For this review, take the finished solid that the model builds, in its own axes (mm). Give positions to 0.01 mm unless a question says otherwise; leave off trailing zeros. Order: outer loops, then holes, each group sorted by start corner. A loop starts at its lowest first (then second) coordinate and runs counter-clockwise, first axis right, second up.
Item 1: Consider section B-B (x = 2.5). Give the boundary of the cut face in (y, z).
Item 2: For probe 1 along X at (y, z) = (-22, 2.5); probe 2 along X at (y, z) = (-23, 2); probe 3 along X at (y, z) = (2.5, 11.75), list the stretches that pass through material, from the lowest coordinate up.
Item 3: Consider section C-C (y = -12). Give the boundary of the cut face in (x, z).
Item 4: Consider section A-A (y = 4.5). Give the boundary of the cut face in (x, z).
Item 5: Consider section D-D (z = 3.5). Give the boundary of the cut face in (x, y) (1 decimal), plus the area to 3 significant figures.
Item 6: For P1, Ø4, axis at y = -10.5, z = 9.5, coming from the -X side; P2, Ø12, axis at x = -30.5, y = -16.5, coming from the +Z side; P3, Ø1.5, axis at x = 10.5, z = 11, coming from the +Y side; P4, Ø1.5, axis at y = 8.5, z = 4.5, coming from the -X side, all flat-tipped, find the tip position at first contact; note any pin that passes through.
Item 7: The part is to be moulded in two halves that separate along X. For faces 1 (the cylindrical face through (1.378, -16.014, 6.261)), 2 (the cylindrical face through (14.928, 7.509, 6.261)), 3 (the flat face through (7, 11, 0)), say which applies: released by +X, released by -X, zero draft, split by the parting line, or undercut.
```python
from build123d import *

# Parameters (mm, degrees)
F0_R     = 10.9982
F0_R_2   = 13.97
F1_DEPTH = 12.7


with BuildPart() as f1:
    # F0 (on Top) → F1 (new body)
    with BuildSketch(Plane.XY):
        with BuildLine():
            ThreePointArc((13.97, 32.0970378816), (12.2885629968, 38.7417440057), (7.6490093808, 43.7869290484))
            ThreePointArc((7.6490093808, 43.7869290484), (0, 44.45), (-7.6490093808, 43.7869290484))
            ThreePointArc((-7.6490093808, 43.7869290484), (-13.7655856932, 34.4781196782), (-11.1311920138, 23.6556242351))
            ThreePointArc((-11.1311920138, 23.6556242351), (-0.5487801971, 18.1378208443), (10.4341459432, 22.8078237902))
            ThreePointArc((10.4341459432, 22.8078237902), (13.0561464228, 27.1273356182), (13.97, 32.0970378816))
        make_face()
        with Locations((0, 32.0970378816)):
            Circle(F0_R, mode=Mode.SUBTRACT)
        with BuildLine():
            ThreePointArc((-7.6490093808, 43.7869290484), (0, 44.45), (7.6490093808, 43.7869290484))
            ThreePointArc((7.6490093808, 43.7869290484), (0, 46.0670378816), (-7.6490093808, 43.7869290484))
        make_face()
        with BuildLine():
            ThreePointArc((36.5141532997, -25.3479606439), (40.1954437919, -20.8685438007), (41.7410377882, -15.2803227832))
            ThreePointArc((41.7410377882, -15.2803227832), (39.4500705459, -20.4815632685), (36.5141532997, -25.3479606439))
        make_face()
        with BuildLine():
            ThreePointArc((36.5141532997, -25.3479606439), (39.4500705459, -20.4815632685), (41.7410377882, -15.2803227832))
            ThreePointArc((41.7410377882, -15.2803227832), (41.7603955997, -14.856098108), (41.7668501917, -14.4314810592))
            ThreePointArc((41.7668501917, -14.4314810592), (37.8325982415, -4.7132167552), (28.245782034, -0.4686962295))
            ThreePointArc((28.245782034, -0.4686962295), (15.8040282066, -7.2667674687), (15.7145912135, -21.4443205685))
            ThreePointArc((15.7145912135, -21.4443205685), (25.2199657431, -28.1617602457), (36.5141532997, -25.3479606439))
        make_face()
        with Locations((27.7968501917, -14.4314810592)):
            Circle(F0_R, mode=Mode.SUBTRACT)
        with BuildLine():
            ThreePointArc((-20.0335070466, -2.8032077223), (-36.5219312191, -5.6152601432), (-38.4948294602, -22.2249995463))
            ThreePointArc((-38.4948294602, -22.2249995463), (-24.9413525406, -29.134012338), (-13.1134053752, -19.5668361497))
            ThreePointArc((-13.1134053752, -19.5668361497), (-12.5992608684, -17.4305143709), (-12.4264543073, -15.24))
            ThreePointArc((-12.4264543073, -15.24), (-14.4790033796, -7.9506061031), (-20.0335070466, -2.8032077223))
        make_face()
        with Locations((-26.3964543073, -15.24)):
            Circle(F0_R, mode=Mode.SUBTRACT)
        with BuildLine():
            ThreePointArc((10.4341459432, 22.8078237902), (-0.5487801971, 18.1378208443), (-11.1311920138, 23.6556242351))
            ThreePointArc((-11.1311920138, 23.6556242351), (-12.8966882758, 9.5225930629), (-20.0335070466, -2.8032077223))
            ThreePointArc((-20.0335070466, -2.8032077223), (-14.4790033796, -7.9506061031), (-12.4264543073, -15.24))
            ThreePointArc((-12.4264543073, -15.24), (-12.5992608684, -17.4305143709), (-13.1134053752, -19.5668361497))
            ThreePointArc((-13.1134053752, -19.5668361497), (1.5922377479, -16.0274926586), (15.7145912135, -21.4443205685))
            ThreePointArc((15.7145912135, -21.4443205685), (15.8040282066, -7.2667674687), (28.245782034, -0.4686962295))
            ThreePointArc((28.245782034, -0.4686962295), (14.7899139444, 7.6877788952), (10.4341459432, 22.8078237902))
        make_face()
        Circle(F0_R_2, mode=Mode.SUBTRACT)
        with Locations((0, 32.0970378816)):
            Circle(F0_R)
        Circle(F0_R_2)
        Circle(F0_R, mode=Mode.SUBTRACT)
    extrude(amount=F1_DEPTH)


solid = f1.part
```
Resolved:
1. outline: (-16.1, 0) - (-10.71, 0) - (-10.71, 12.7) - (-16.1, 12.7) - close; (10.71, 0) - (45.84, 0) - (45.84, 12.7) - (10.71, 12.7) - close
2. probe 1: x = -38.62 to -35.07, -17.72 to -14.17, 16.05 to 19.82, 35.78 to 39.54
2. probe 2: x = -38.01 to -34.19, -18.6 to -14.78, 16.76 to 20.9, 34.69 to 38.83
2. probe 3: x = -16.14 to -10.71, 10.71 to 20.49
3. outline: (-39.99, 0) - (-36.91, 0) - (-36.91, 12.7) - (-39.99, 12.7) - close; (-15.89, 0) - (17.07, 0) - (17.07, 12.7) - (-15.89, 12.7) - close; (38.52, 0) - (41.55, 0) - (41.55, 12.7) - (38.52, 12.7) - close
4. outline: (-15.03, 0) - (-10.04, 0) - (-10.04, 12.7) - (-15.03, 12.7) - close; (10.04, 0) - (17.79, 0) - (17.79, 12.7) - (10.04, 12.7) - close
5. outline: (-20, -2.8) arc R14 ccw (long way) to (-13.1, -19.6) arc R25.5 cw to (15.7, -21.4) arc R14 ccw (long way) to (28.2, -0.5) arc R21.6 cw to (10.4, 22.8) arc R14 ccw (long way) to (-11.1, 23.7) arc R35.8 cw to start; hole circle Ø22 at (-26.4, -15.2); hole circle Ø22 at (0, 0); hole circle Ø22 at (27.8, -14.4)
5. area: 1,800 mm2
6. P1: stops at x = -40.1
6. P2: passes through
6. P3: stops at y = 42.1
6. P4: stops at x = -13.55
7. face 1: undercut
7. face 2: released by +X
7. face 3: zero draft
